Verification items for the finished model (mm, model axes). Face numbers are marked on the shaded views. A direction names the side the tool comes from. Round coordinates to 2 decimals unless told otherwise and drop trailing zeros. Write each loop counter-clockwise with the first axis right and the second up, starting at its lowest first coordinate (ties: lowest second). Pieces come first, ordered by that corner, then holes. Notation, with made-up numbers: (29, 89) - (37, 89) arc R22 cw to (37, 107) - close; hole circle Ø7 at (32, 23). An arc over 180 degrees is marked (long way). Answer as a JSON object with one key per item and string values. Group by question number.
1) Section check A-A (z = 0). Enter the section's corners in (x, y).
2) Thickness scan on line 1 (Y direction, x = -1.6, z = 0.85); line 2 (X direction, y = -1.25, z = -0.25); line 3 (Y direction, x = -0.1, z = 0.65). Record the ranges inside material, lowest first.
3) Section check C-C (y = -5). Enter the section's corners in (x, z), then the cut area to 3 significant figures.
4) Section check D-D (z = -2.4). Enter the section's corners in (x, y).
5) Section check B-B (y = 1). Enter the section's corners in (x, z).
6) Set-up check for the marked faces 1 and 2: record each of +Z, -Z, +X, -X, +Y, -Y from which the full face is reachable in a straight line by a thin tool's end or side.
7) Go/stop test with flat-tipped pins: pin 1 Ø1 at (x, y) = (-0.5, -4) entering from +Z; pin 2 Ø1 at (y, z) = (-4, -1.5) entering from -X. Record where each tip stops, or that it passes through.
```python
from build123d import *

# Parameters (mm, degrees)
SKETCH_2_R          = 5
CUT_EXTRUDE_1_DEPTH = 5.3


with BuildPart() as part:
    # Эскиз1 → Повернуть1 (revolve)
    with BuildSketch(Plane.XY, mode=Mode.PRIVATE) as revolve_1_sk:
        with BuildLine():
            Line((3, 3.550626861), (3, 0))
            Line((3, 0), (2, 0))
            Line((2, 0), (2, -6.5705))
            Line((2, -6.5705), (1.5705, -7))
            Line((1.5705, -7), (0, -7))
            Line((0, -7), (0, 5.3))
            ThreePointArc((0, 5.3), (0.145773797, 5.259622996), (0.25, 5.15))
            ThreePointArc((0.25, 5.15), (1.811111153, 4.670317349), (3, 3.550626861))
        make_face()
    revolve(revolve_1_sk.sketch.rotate(Axis((0, -7, 0), (0, 1, 0)), 270), axis=Axis((0, -7, 0), (0, 1, 0)))

    # Эскиз2 → Вырез-Вытянуть1 (cut)
    with BuildSketch(Plane(origin=(0, 0, 0), x_dir=(1, 0, 0), z_dir=(0, 1, 0))):
        Circle(SKETCH_2_R)
        Polygon((-2.5, 1.443375673), (-2.5, -1.443375673), (0, -2.886751346), (2.5, -1.443375673), (2.5, 1.443375673), (0, 2.886751346), align=None, mode=Mode.SUBTRACT)
    extrude(amount=CUT_EXTRUDE_1_DEPTH, mode=Mode.SUBTRACT)


solid = part.part
```
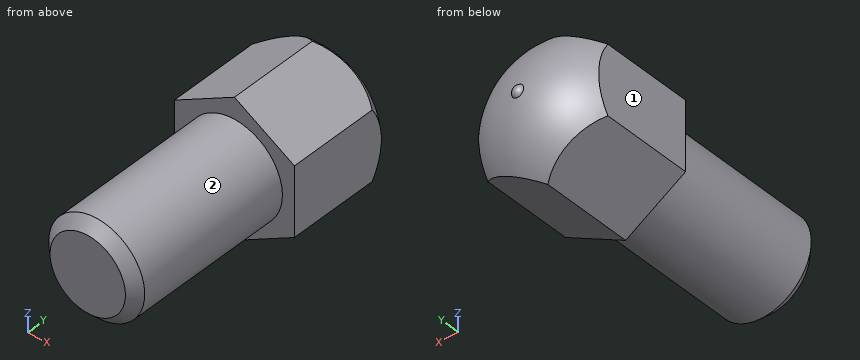
Returned:
{
 "1": {"outline": "(-2.5, 0) - (-2, 0) - (-2, -6.57) - (-1.57, -7) - (1.57, -7) - (2, -6.57) - (2, 0) - (2.5, 0) - (2.5, 4.15) arc R3.6 ccw to (0.25, 5.15) arc R0.28 ccw to (-0.25, 5.15) arc R3.6 ccw to (-2.5, 4.15) - close"},
 "2": {"line 1": "-6.76 to 4.67", "line 2": "-1.98 to 1.98", "line 3": "-7 to 5.1"},
 "3": {"outline": "circle Ø4 at (0, 0)", "area": "12.6 mm2"},
 "4": {"outline": "(-0.84, 0) - (0.84, 0) - (0.84, 4.11) arc R2.69 ccw to (-0.84, 4.11) - close"},
 "5": {"outline": "(-2.5, -1.44) - (0, -2.89) - (2.5, -1.44) - (2.5, 1.44) - (0, 2.89) - (-2.5, 1.44) - close"},
 "6": {"face 1": "+Z, -Z, -X, +Y, -Y", "face 2": "-Y"},
 "7": {"pin 1": "z = 2", "pin 2": "x = -1.73"}
}
